from build123d import *

# Parameters (mm, degrees)
SWEEP1_PROFILE_R   = 13.97
SHELL1_T           = -3.175
CUT_EXTRUDE1_START = -13.208
SKETCH28_R         = 10.795
CUT_EXTRUDE1_DEPTH = 13.208


with BuildPart() as part:
    # Sweep1: sweep along a path in Sketch1
    with BuildLine(Plane.XY) as sweep1_path:
        Line((0, 0), (0, 13.97))
        ThreePointArc((0, 13.97), (5.207641431, 26.542358569), (17.78, 31.75))
        Line((17.78, 31.75), (31.75, 31.75))
    # Sweep1 profile (on start of the path) → Sweep1 (sweep)
    with BuildSketch(Plane.ZX):
        Circle(SWEEP1_PROFILE_R)
    sweep(path=sweep1_path.line)

    # Shell1
    shell1_openings = [part.faces().sort_by_distance(p)[0] for p in [
        (31.75, 31.75, 0),
    ]]
    offset(amount=SHELL1_T, openings=shell1_openings, kind=Kind.INTERSECTION)

    # Sketch28 → Cut-Extrude1 (cut)
    with BuildSketch(Plane.XZ.offset(CUT_EXTRUDE1_START)):
        with Locations(Location((0, 0, 0), (0, 0, 180))):
            Circle(SKETCH28_R)
    extrude(amount=CUT_EXTRUDE1_DEPTH, mode=Mode.SUBTRACT)


solid = part.part
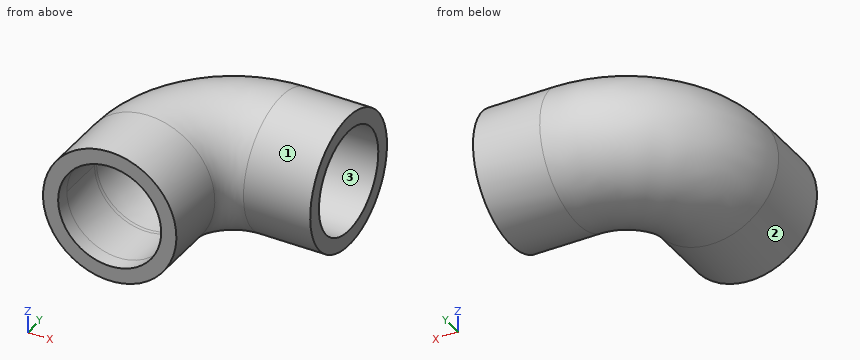
Design review of the part built by this model. Coordinates are the model's own, in mm. Face numbers are marked on the shaded views. Round coordinates to 2 decimals unless told otherwise and drop trailing zeros. Loops run counter-clockwise (first coordinate to the right, second up) from the corner with the lowest first, then second, coordinate; pieces in that order, holes last. Notation, with made-up numbers: M 26.5,36 L 70.5,36 A29 ccw 70.5,66 Z; hole C 16.25,-1.5 d9. An arc over 180 degrees is marked long. Answer as a JSON object with one key per item and string values.
Item 1: We need section B-B on z = -12. Give the boundary of the cut face in (x, y).
Answer sheet:
{"outline": "M -7.15,0 L 7.15,0 L 7.15,13.97 A10.63 cw 17.78,24.6 L 31.75,24.6 L 31.75,38.9 L 17.78,38.9 A24.93 ccw -7.15,13.97 Z"}
Item 2: Clearance check with flat-ended pins moving along their axes: P1, Ø4, axis at y = 19.5, z = -11, coming from the -X side; P2, Ø13, axis at x = 0, z = 0, coming from the -Y side; P3, Ø6, axis at x = -4, z = 1, coming from the +Y side; P4, Ø10, axis at x = 14, z = -3, coming from the +Y side. State where each tip first meets the part, or that it passes through.
Answer sheet:
{"P1": "stops at x = -10.18", "P2": "stops at y = 29.04", "P3": "stops at y = 39.54", "P4": "stops at y = 45.72"}
Item 3: The part is to be moulded in two halves that separate along Y. For the marked faces 1, 2 and 3, say which applies: pulls with the +Y half, pulls with the -Y half, needs draft (parallel to the pull), parting line crosses it, or undercut.
Answer sheet:
{"face 1": "parting line crosses it", "face 2": "needs draft", "face 3": "undercut"}
Item 4: We need section A-A on z = 5. Give the boundary of the cut face in (x, y), and give its area (3 significant figures).
Answer sheet:
{"outline": "M -13.04,0 L -9.57,0 L -9.57,13.97 A27.35 cw 17.78,41.32 L 31.75,41.32 L 31.75,44.79 L 17.78,44.79 A30.82 ccw -13.04,13.97 Z; M 9.57,0 L 13.04,0 L 13.04,13.97 A4.74 cw 17.78,18.71 L 31.75,18.71 L 31.75,22.18 L 17.78,22.18 A8.21 ccw 9.57,13.97 Z", "area": "389 mm^2"}
Item 5: Wall thickness on L1, parallel to X at y = 10.5, z = 0 (3 decimals); L2, parallel to Z at x = 28, y = 39; L3, parallel to Z at x = 27, y = 28.5: over which ranges is each line inside the solid? List them lowest first. Write a range as from..to.
Answer sheet:
{"L1": "x = -13.97..-10.795, 10.795..13.97", "L2": "z = -11.94..-8, 8..11.94", "L3": "z = -13.59..-10.29, 10.29..13.59"}
Item 6: We need section C-C on z = -3.5. Give the boundary of the cut face in (x, y).
Answer sheet:
{"outline": "M -13.52,0 L -10.21,0 L -10.21,13.97 A27.99 cw 17.78,41.96 L 31.75,41.96 L 31.75,45.27 L 17.78,45.27 A31.3 ccw -13.52,13.97 Z; M 10.21,0 L 13.52,0 L 13.52,13.97 A4.26 cw 17.78,18.23 L 31.75,18.23 L 31.75,21.54 L 17.78,21.54 A7.57 ccw 10.21,13.97 Z"}
